Geometry: see drawing. Coordinates: mm, zero at the bounding-box minimum. A direction names the side the tool comes from. Give positions to 0.01 mm unless a question says otherwise; leave off trailing zeros. Loops run counter-clockwise (first coordinate to the right, second up) from the corner with the lowest first, then second, coordinate; pieces in that order, holes last. Notation, with made-up numbers: M 41,6.25 L 99,6.25 A16 ccw 99,29.25 Z; hole C 58,-3.5 d5. An arc over 180 degrees is marked long. Put each result on its own line as item: value.
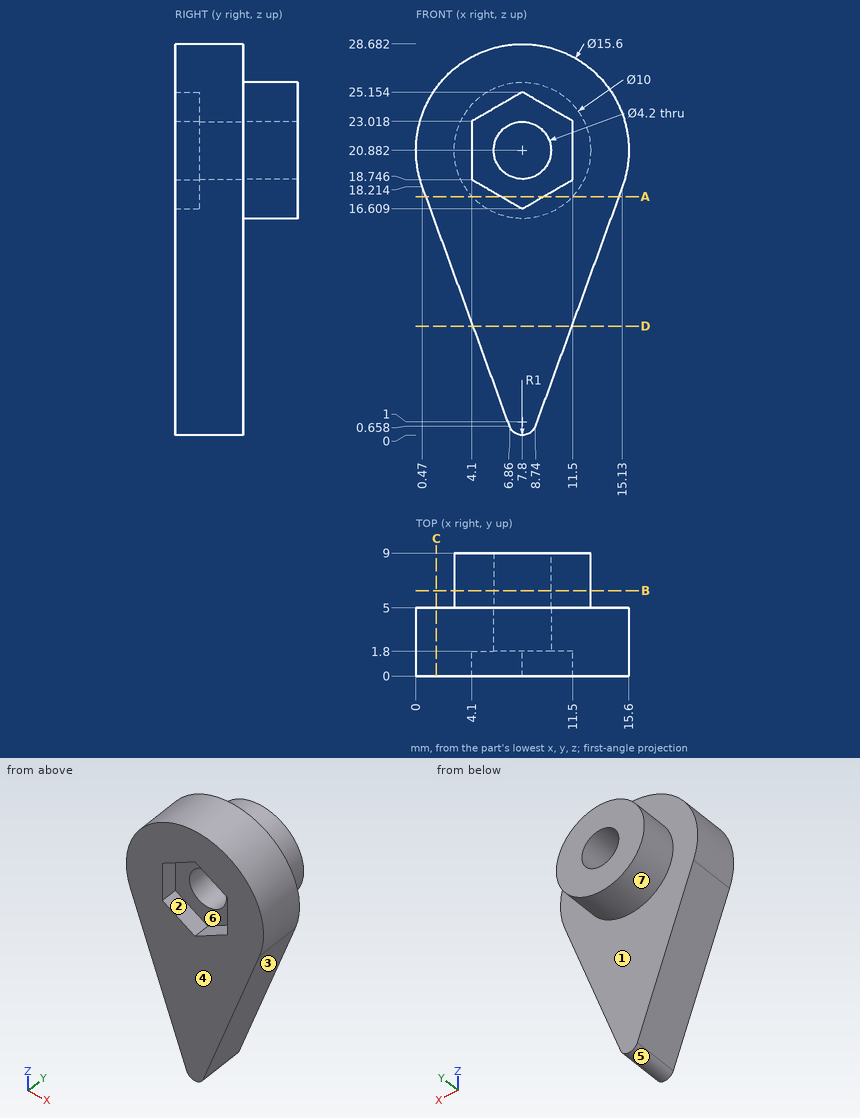
1. Section query A-A (z = 17.5). Output: boundary loops of the cut face in (x, y).
Found:
outline: M 0.73,0 L 6.26,0 L 6.26,1.8 L 9.34,1.8 L 9.34,0 L 14.87,0 L 14.87,5 L 11.48,5 L 11.48,9 L 4.12,9 L 4.12,5 L 0.73,5 Z
2. Contact query for flat-ended pins moving along their axis: P1, Ø3, axis at x = 7, y = 7, coming from the +Z side; P2, Ø3, axis at y = 6, z = 5, coming from the +X side; P3, Ø0.5, axis at y = 1, z = 21.5, coming from the -X side. Output: stop coordinate, or through.
Found:
P1: z = 25.88
P2: x = 10.73
P3: x = 0.01
3. Access query for the marked faces 1, 2 and 3. Directions: +Z, -Z, +X, -X, +Y, -Y. A direction counts if a zero-diameter tool reaches every point of the face in a straight line with its end or side. Return the directions, or none.
Found:
face 1: +Y
face 2: -Y
face 3: -Z, +X, +Y, -Y
4. Section query D-D (z = 8). Output: boundary loops of the cut face in (x, y), plus the area to 3 significant figures.
Found:
outline: M 4.19,0 L 11.41,0 L 11.41,5 L 4.19,5 Z
area: 36.1 mm^2
5. Material intervals for line 1 (X direction, y = 7.5, z = 20.75) (1 decimal); line 2 (Y direction, x = 6.5, z = 13.25); line 3 (Z direction, x = 7.8, y = 6.85), sorted ascending. Write a range as from..to.
Found:
line 1: 2.8..5.7, 9.9..12.8
line 2: 0..5
line 3: 15.88..18.78, 22.98..25.88
6. Section query B-B (y = 6.25). Output: boundary loops of the cut face in (x, z).
Found:
outline: C 7.8,20.88 d10; hole C 7.8,20.88 d4.2
7. Section query C-C (x = 1.5). Output: boundary loops of the cut face in (y, z) (1 decimal).
Found:
outline: M 0,15.4 L 5,15.4 L 5,25.5 L 0,25.5 Z
8. Draft query along Z for the marked faces 4, 5, 6 and 7. Return one class per face: pulls with the +Z half, pulls with the -Z half, needs draft (parallel to the pull), parting line crosses it, or undercut.
Found:
face 4: needs draft
face 5: pulls with the -Z half
face 6: undercut
face 7: parting line crosses it
